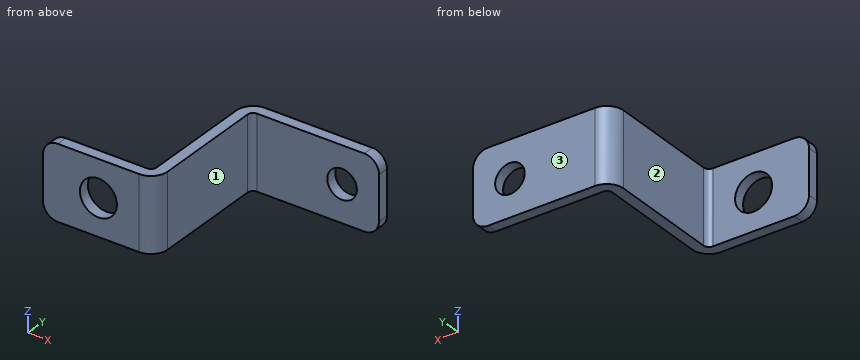
```python
from build123d import *

# Parameters (mm, degrees)
BASE_FLANGE1_DEPTH = 10
SKETCH6_R          = 2.5
CUT_EXTRUDE1_DEPTH = 39.474017206
SKETCH7_R          = 2
CUT_EXTRUDE2_DEPTH = 40.198214245
FILLET1_R          = 2


# Sheet-metal steps are written as plain solids
with BuildPart() as part:
    # Sketch1 → Base-Flange1 (new body)
    with BuildSketch(Plane.XY):
        with BuildLine():
            Line((0, 0), (13, 0))
            ThreePointArc((13, 0), (13.530330086, 0.219669914), (13.75, 0.75))
            Line((13.75, 0.75), (13.75, 15.75))
            ThreePointArc((13.75, 15.75), (14.409009742, 17.340990258), (16, 18))
            Line((16, 18), (32.5, 18))
            Line((32.5, 18), (32.5, 16.5))
            Line((32.5, 16.5), (16, 16.5))
            ThreePointArc((16, 16.5), (15.469669914, 16.280330086), (15.25, 15.75))
            Line((15.25, 15.75), (15.25, 0.75))
            ThreePointArc((15.25, 0.75), (14.590990258, -0.840990258), (13, -1.5))
            Line((13, -1.5), (0, -1.5))
            Line((0, -1.5), (0, 0))
        make_face()
    extrude(amount=BASE_FLANGE1_DEPTH)

    # Sketch6 → Cut-Extrude1 (cut, through all)
    with BuildSketch(Plane(origin=(0, 0, 0), x_dir=(1, 0, 0), z_dir=(0, 1, 0))):
        with Locations(Location((7.5, -5, 0), (0, 0, 270))):
            Circle(SKETCH6_R)
    extrude(amount=-CUT_EXTRUDE1_DEPTH, mode=Mode.SUBTRACT)

    # Sketch7 → Cut-Extrude2 (cut, through all)
    with BuildSketch(Plane(origin=(0, 18, 0), x_dir=(1, 0, 0), z_dir=(0, 1, 0))):
        with Locations(Location((27.5, -5, 0), (0, 0, 270))):
            Circle(SKETCH7_R)
    extrude(amount=-CUT_EXTRUDE2_DEPTH, mode=Mode.SUBTRACT)

    # Fillet1
    fillet1_edges = [part.edges().sort_by_distance(p)[0] for p in [
        (0, -0.75, 0),
        (32.5, 17.25, 0),
        (0, -0.75, 10),
        (32.5, 17.25, 10),
    ]]
    fillet(fillet1_edges, radius=FILLET1_R)


solid = part.part
```
Could you check a few things on this model? Use its own coordinates, in mm. Face numbers are marked on the shaded views. A direction names the side the tool comes from. Round coordinates to 2 decimals unless told otherwise and drop trailing zeros. Loops run counter-clockwise (first coordinate to the right, second up) from the corner with the lowest first, then second, coordinate; pieces in that order, holes last. Notation, with made-up numbers: (54, 16) - (113, 16) arc R27 ccw to (113, 49) - close; hole circle Ø11 at (34, 89.25). An arc over 180 degrees is marked (long way). Answer in a Markdown table with one row per item. Add a question column.
(1) If we section it at B-B (x = 7.5): Please give me the cut outline in (y, z).
(2) For the marked faces 1, 2 and 3, which set-ups out of +Z, -Z, +X, -X, +Y, -Y let a thin tool reach every point of the face, with its end or its side?
(3) I'm going to push flat-ended pins straight in: pin 1 (1 mm diameter, centred on y = 12.5, z = 2, fed in from +X); pin 2 (1.5 mm diameter, centred on y = 8.5, z = 2, fed in from -X); pin 3 (3 mm diameter, centred on x = 20.5, z = 7, fed in from -Y); pin 4 (2.5 mm diameter, centred on x = 27.5, z = 5, fed in from +Y). Where does each tip first touch, or does it pass through?
(4) If we section it at A-A (z = 5): Please give me the cut outline in (x, y).
(5) If we section it at C-C (x = 27.5): Please give me the cut outline in (y, z).
(6) I need wall thicknesses on line 1 along Y through (x, z) = (5.5, 8.25); line 2 along Y through (x, z) = (23, 7.75); line 3 along X through (y, z) = (11, 0.5). Which ranges of each line are inside material? Lowest first, please.
(7) If we section it at D-D (z = 3.5): Please give me the cut outline in (x, y).
Model answer:
| question | item | result |
|---|---|---|
| 1 | outline | (-1.5, 0) - (0, 0) - (0, 2.5) - (-1.5, 2.5) - close; (-1.5, 7.5) - (0, 7.5) - (0, 10) - (-1.5, 10) - close |
| 2 | face 1 | +Z, -Z, +X, -Y |
| 2 | face 2 | +Z, -Z, -X, +Y |
| 2 | face 3 | +Z, -Z, +X, -X, +Y |
| 3 | pin 1 | stops at x = 15.25 |
| 3 | pin 2 | stops at x = 13.75 |
| 3 | pin 3 | stops at y = 16.5 |
| 3 | pin 4 | passes through |
| 4 | outline | (0, -1.5) - (5, -1.5) - (5, 0) - (0, 0) - close; (10, -1.5) - (13, -1.5) arc R2.25 ccw to (15.25, 0.75) - (15.25, 15.75) arc R0.75 cw to (16, 16.5) - (25.5, 16.5) - (25.5, 18) - (16, 18) arc R2.25 ccw to (13.75, 15.75) - (13.75, 0.75) arc R0.75 cw to (13, 0) - (10, 0) - close; (29.5, 16.5) - (32.5, 16.5) - (32.5, 18) - (29.5, 18) - close |
| 5 | outline | (16.5, 0) - (18, 0) - (18, 3) - (16.5, 3) - close; (16.5, 7) - (18, 7) - (18, 10) - (16.5, 10) - close |
| 6 | line 1 | y = -1.5 to 0 |
| 6 | line 2 | y = 16.5 to 18 |
| 6 | line 3 | x = 13.75 to 15.25 |
| 7 | outline | (0, -1.5) - (5.5, -1.5) - (5.5, 0) - (0, 0) - close; (9.5, -1.5) - (13, -1.5) arc R2.25 ccw to (15.25, 0.75) - (15.25, 15.75) arc R0.75 cw to (16, 16.5) - (26.18, 16.5) - (26.18, 18) - (16, 18) arc R2.25 ccw to (13.75, 15.75) - (13.75, 0.75) arc R0.75 cw to (13, 0) - (9.5, 0) - close; (28.82, 16.5) - (32.5, 16.5) - (32.5, 18) - (28.82, 18) - close |
